Drawing for the job (mm, zero at the part's lowest x, y, z). A direction names the side the tool comes from. Coordinates: 2 decimals unless noted, no trailing zeros. Order: outer loops, then holes, each group sorted by start corner. A loop starts at its lowest first (then second) coordinate and runs counter-clockwise, first axis right, second up.
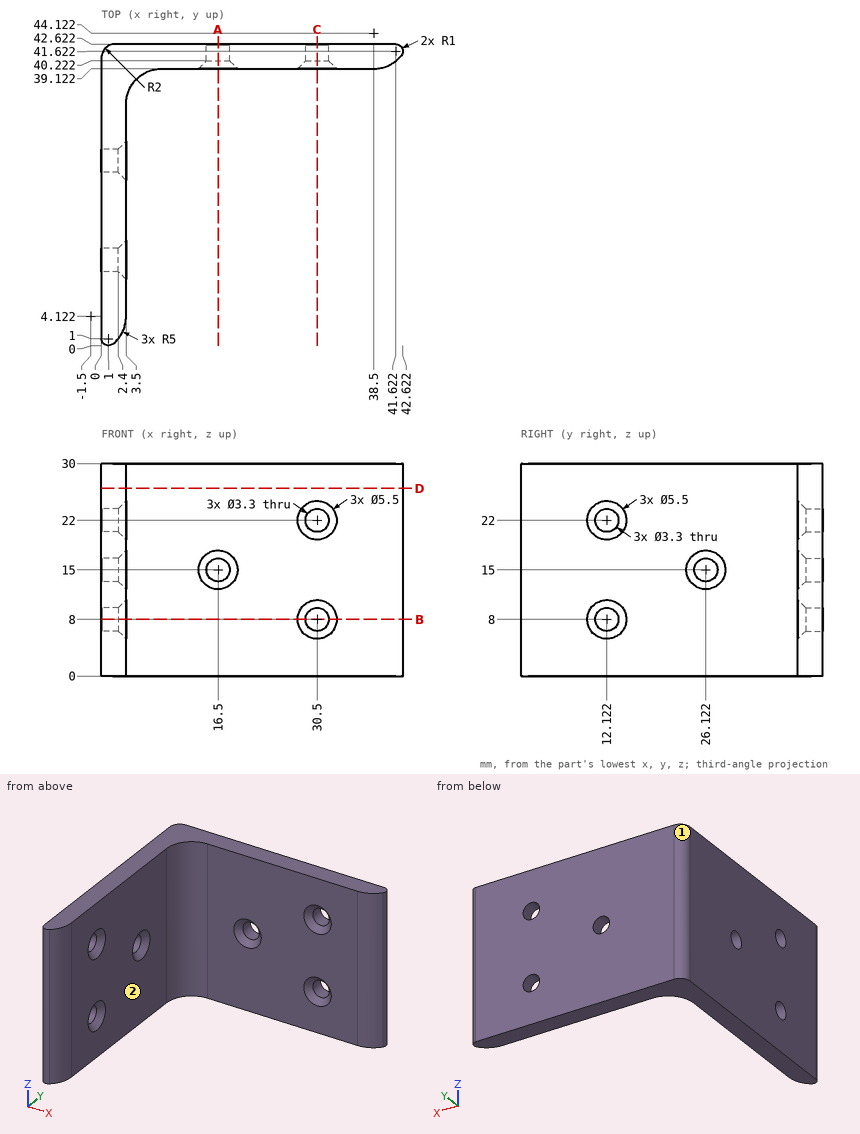
1) Slice it at B-B (z = 8). Give the number of separate pieces and of enclosed holes in the cut face, plus the area to 3 significant figures.
2) Drill centre lines: probe 1 along Z at (x, y) = (30.5, 41.65); probe 2 along Z at (x, y) = (30, 40) (1 decimal); probe 3 along Y at (x, z) = (12, 5.25). Where is each one in solid material? Low to high.
3) Slice it at D-D (z = 26.5). List the corners of the cut face in (x, y) (1 decimal), plus the area to 3 significant figures.
4) Slice it at A-A (x = 16.5). List the corners of the cut face in (y, z).
5) Pin check, flat tips, straight feed: P1, Ø4, axis at y = 14, z = 6, coming from the +X side; P2, Ø5, axis at x = 4.5, z = 13.5, coming from the -Y side; P3, Ø15, axis at x = 23.5, z = 21, coming from the -Y side. Stop position of each tip, or through.
6) Slice it at C-C (x = 30.5). List the corners of the cut face in (y, z).
7) Which spindle directions (+Z, -Z, +X, -X, +Y, -Y) get a long thin tool onto all of the face, cutting with end or side? Do the marked faces 1 and 2. Say none if no direction does.
Worked out:
1. separate pieces: 3
1. enclosed holes: 0
1. area: 259 mm2
2. probe 1: z = 0 to 6.35, 9.65 to 20.35, 23.65 to 30
2. probe 2: z = 0 to 6.2, 9.8 to 20.2, 23.8 to 30
2. probe 3: y = 39.12 to 42.62
3. outline: (0, 1) arc R1 ccw to (1.6, 0.2) arc R5 ccw to (3.5, 4.1) - (3.5, 34.1) arc R5 cw to (8.5, 39.1) - (38.5, 39.1) arc R5 ccw to (42.4, 41) arc R1 ccw to (41.6, 42.6) - (2, 42.6) arc R2 ccw to (0, 40.6) - close
3. area: 285 mm2
4. outline: (39.12, 0) - (42.62, 0) - (42.62, 13.35) - (40.22, 13.35) - (39.12, 12.25) - close; (39.12, 17.75) - (40.22, 16.65) - (42.62, 16.65) - (42.62, 30) - (39.12, 30) - close
5. P1: stops at x = 3.5
5. P2: stops at y = 0.55
5. P3: stops at y = 39.12
6. outline: (39.12, 0) - (42.62, 0) - (42.62, 6.35) - (40.22, 6.35) - (39.12, 5.25) - close; (39.12, 10.75) - (40.22, 9.65) - (42.62, 9.65) - (42.62, 20.35) - (40.22, 20.35) - (39.12, 19.25) - close; (39.12, 24.75) - (40.22, 23.65) - (42.62, 23.65) - (42.62, 30) - (39.12, 30) - close
7. face 1: +Z, -Z, -X, +Y
7. face 2: +Z, -Z, +X, -Y
